```python
from build123d import *

# Parameters (mm, degrees)
F1_DEPTH = 1000
F3_D     = 8
F3_DEPTH = 10
F3_TIP   = 2.4034424761


with BuildPart() as f1:
    # F0 (on Top) → F1 (new body)
    with BuildSketch(Plane.XY):
        with BuildLine():
            Line((20, 0), (-20, 0))
            ThreePointArc((-20, 0), (0, -20), (20, 0))
        make_face()
    extrude(amount=F1_DEPTH)

    # F3
    with Locations(Plane(origin=(0, 0, 0), x_dir=(-1, 0, 0), z_dir=(0, 1, 0))):
        with Locations((-10, 280), (10, 280), (-10, 120), (10, 120)):
            Hole(F3_D / 2, depth=F3_DEPTH)
            with Locations((0, 0, -(F3_DEPTH + F3_TIP / 2))):  # 118° drill point
                Cone(0, F3_D / 2, F3_TIP, mode=Mode.SUBTRACT)


solid = f1.part
```
Part model, mm, in its own coordinate system. Round coordinates to 2 decimals unless told otherwise and drop trailing zeros. Loops run counter-clockwise (first coordinate to the right, second up) from the corner with the lowest first, then second, coordinate; pieces in that order, holes last.
1. Flat gauge pins, fed straight in: pin 1 (6 mm diameter, centred on x = -10.5, z = 650, fed in from -Y); pin 2 (1.5 mm diameter, centred on x = -2, z = 242.5, fed in from +Y); pin 3 (2 mm diameter, centred on y = -13, z = 252, fed in from -X); pin 4 (6 mm diameter, centred on y = -13, z = 211, fed in from +X). Where does each tip first touch, or does it go through?
Solutions:
pin 1: stops at y = -18.54
pin 2: stops at y = 0
pin 3: stops at x = -16
pin 4: stops at x = 17.32
2. Drill centre lines: line 1 along Z through (x, y) = (10, -3.75); line 2 along X through (y, z) = (-5.5, 279.5); line 3 along X through (y, z) = (-5.25, 280). Where is each one in solid material? Low to high.
Solutions:
line 1: z = 0 to 116, 124 to 276, 284 to 1000
line 2: x = -19.23 to -13.97, -6.03 to 6.03, 13.97 to 19.23
line 3: x = -19.3 to -14, -6 to 6, 14 to 19.3
3. Slice it at A-A (z = 258.5). Give the cut face in (x, y).
Solutions:
outline: (-20, 0) arc R20 ccw to (20, 0) - close
